Check sheet for the modelled part. Datum: model origin and axes. Units: mm. A direction names the side the tool comes from. Give positions to 0.01 mm unless a question says otherwise; leave off trailing zeros. Loops run counter-clockwise (first coordinate to the right, second up) from the corner with the lowest first, then second, coordinate; pieces in that order, holes last.
```python
from build123d import *

# Parameters (mm, degrees)
SKETCH_R  = 4
PAD_DEPTH = 5.5


with BuildPart() as part:
    # Sketch → Pad (new body)
    with BuildSketch(Plane.XZ):
        with BuildLine():
            Line((-29, 8), (35, 8))
            ThreePointArc((35.281785, 5.026705), (36.493309, 6.641524), (35, 8))
            Line((9, 0), (35.281785, 5.026705))
            ThreePointArc((-8.774964, -2), (1.00631, -8.943564), (9, 0))
            Line((-8.774964, -2), (-13.249792, -2))
            ThreePointArc((-13.249792, -2), (-14.193003, 0.183946), (-16.429538, 0.99461))
            Line((-33, 0), (-16.429538, 0.99461))
            Line((-29, 8), (-33, 0))
        make_face()
        Circle(SKETCH_R, mode=Mode.SUBTRACT)
    extrude(amount=PAD_DEPTH)


solid = part.part
```
(1) Access from +Z, -Z, +X, -X, +Y, -Y to the whole of each face (thin tool, end or side, straight path). Record for faces 1 (the face through (36.496, -2.712, 6.611)), 2 (the face through (-14.17, -2.71, 0.16)).
(2) Gauge pin test, flat ends, axial feed: pin 1 Ø2 at (x, y) = (-20, -1.5) entering from -Z; pin 2 Ø3 at (x, y) = (-23.5, -3) entering from -Z; pin 3 Ø3 at (y, z) = (-2, -3) entering from -X. Record the tip position at first contact, or that the pin passes through.
(3) Section check C-C on z = 2. Record the boundary of the cut face in (x, y), plus the area to 3 significant figures.
(4) Material ranges on line 1 (Z direction, x = 0, y = -1.65); line 2 (X direction, y = -1.05, z = -3.5); line 3 (X direction, y = -1.4, z = -2.75), recorded low to high.
(5) Section check A-A on x = 0. Record the boundary of the cut face in (y, z).
(6) Section check D-D on x = -12.5. Record the boundary of the cut face in (y, z), plus the area to 3 significant figures.
(7) Release check for a two-part mould opening along X. For faces 3 (the face through (-31, -3, 4)), 4 (the face through (-11, -3, -2)), 5 (the face through (-0.867, -2.712, -3.905)), 6 (the face through (0.823, -2.712, -8.962)) record: pulls with the +X half, pulls with the -X half, needs draft (parallel to the pull), parting line crosses it, or undercut.
(8) Section check B-B on y = -3.45. Record the boundary of the cut face in (x, z).
Computed values:
1. face 1: +X, +Y, -Y
1. face 2: -Z, +Y, -Y
2. pin 1: stops at z = 0.72
2. pin 2: stops at z = 0.48
2. pin 3: stops at x = -13.29
3. outline: (-32, -5.5) - (-3.46, -5.5) - (-3.46, 0) - (-32, 0) - close; (3.46, -5.5) - (19.46, -5.5) - (19.46, 0) - (3.46, 0) - close
3. area: 245 mm2
4. line 1: z = -9 to -4, 4 to 8
4. line 2: x = -8.29 to -1.94, 1.94 to 8.29
4. line 3: x = -8.57 to -2.9, 2.9 to 8.57
5. outline: (-5.5, -9) - (0, -9) - (0, -4) - (-5.5, -4) - close; (-5.5, 4) - (0, 4) - (0, 8) - (-5.5, 8) - close
6. outline: (-5.5, -2) - (0, -2) - (0, 8) - (-5.5, 8) - close
6. area: 55.0 mm2
7. face 3: pulls with the -X half
7. face 4: needs draft
7. face 5: undercut
7. face 6: parting line crosses it
8. outline: (-33, 0) - (-16.43, 0.99) arc R3 cw to (-13.25, -2) - (-8.77, -2) arc R9 ccw to (9, 0) - (35.28, 5.03) arc R1.5 ccw to (35, 8) - (-29, 8) - close; hole circle Ø8 at (0, 0)
